Geometry check sheet. Reference: the model listing, model coordinates, mm. A direction names the side the tool comes from. Round coordinates to 2 decimals unless told otherwise and drop trailing zeros. Order: outer loops, then holes, each group sorted by start corner. A loop starts at its lowest first (then second) coordinate and runs counter-clockwise, first axis right, second up.
(1) Thickness scan on L1, parallel to X at y = 6.5, z = -5; L2, parallel to X at y = 5.5, z = -21; L3, parallel to Z at x = 78.5, y = 8.25. Record the ranges inside material, lowest first.
(2) Draft check along Z on faces 6 (the face through (-81, 5, 10)), 7 (the face through (1, 10, 20)), 8 (the face through (0, 5, 0)), 9 (the face through (0, 8, 13)). Enter one of: pulls with the +Z half, pulls with the -Z half, needs draft (parallel to the pull), parting line crosses it, or undercut.
(3) Gauge pin test, flat ends, axial feed: P1, Ø12, axis at x = -1, z = -5, coming from the +Y side; P2, Ø5, axis at x = -81, y = 4.5, coming from the -Z side; P3, Ø5, axis at y = 2, z = 18.5, coming from the -X side; P4, Ø6, axis at x = 73.5, z = -32, coming from the +Y side. Record the tip position at first contact, or that the pin passes through.
(4) Cross-section at B-B on y = 3.25. Enter the section's corners in (x, z).
(5) Cross-section at A-A on x = 3.5. Enter the section's corners in (y, z).
(6) Cross-section at C-C on z = 34. Enter the section's corners in (x, y).
(7) Set-up check for faces 1 (the face through (-7.5, 8, 0)), 2 (the face through (-68.5, 5, 29)), 3 (the face through (-68.5, 5, -28)), 4 (the face through (81, 5, -10)), 5 (the face through (81, 5, 10)): record each of +Z, -Z, +X, -X, +Y, -Y from which the full face is reachable in a straight line by a thin tool's end or side.
from build123d import *

# Parameters (mm, degrees)
SALIENTE_EXTRUIR1_DEPTH = 10
CROQUIS3_W              = 15
CROQUIS3_H              = 26
CORTAR_EXTRUIR3_DEPTH   = 5


with BuildPart() as part:
    # Croquis1 → Saliente-Extruir1 (new body)
    with BuildSketch(Plane(origin=(0, 0, 0), x_dir=(1, 0, 0), z_dir=(0, 1, 0))):
        Polygon((93.5, -10), (68.5, -10), (68.5, -47), (-68.5, -47), (-68.5, -10), (-93.5, -10), (-93.5, 10), (-68.5, 10), (-68.5, 47), (68.5, 47), (68.5, 10), (93.5, 10), align=None)
    extrude(amount=SALIENTE_EXTRUIR1_DEPTH)

    # Croquis3 → Cortar-Extruir3 (cut)
    with BuildSketch(Plane(origin=(0, 10, 0), x_dir=(1, 0, 0), z_dir=(0, 1, 0))):
        Rectangle(CROQUIS3_W, CROQUIS3_H)
    extrude(amount=-CORTAR_EXTRUIR3_DEPTH, mode=Mode.SUBTRACT)


solid = part.part
Found:
1. L1: x = -93.5 to -7.5, 7.5 to 93.5
1. L2: x = -68.5 to 68.5
1. L3: z = -10 to 10
2. face 6: pulls with the +Z half
2. face 7: needs draft
2. face 8: undercut
2. face 9: undercut
3. P1: stops at y = 5
3. P2: stops at z = -10
3. P3: stops at x = -68.5
3. P4: passes through
4. outline: (-93.5, -10) - (-68.5, -10) - (-68.5, -47) - (68.5, -47) - (68.5, -10) - (93.5, -10) - (93.5, 10) - (68.5, 10) - (68.5, 47) - (-68.5, 47) - (-68.5, 10) - (-93.5, 10) - close
5. outline: (0, -47) - (10, -47) - (10, -13) - (5, -13) - (5, 13) - (10, 13) - (10, 47) - (0, 47) - close
6. outline: (-68.5, 0) - (68.5, 0) - (68.5, 10) - (-68.5, 10) - close
7. face 1: +Y
7. face 2: +Z, -X, +Y, -Y
7. face 3: -Z, -X, +Y, -Y
7. face 4: -Z, +X, +Y, -Y
7. face 5: +Z, +X, +Y, -Y
